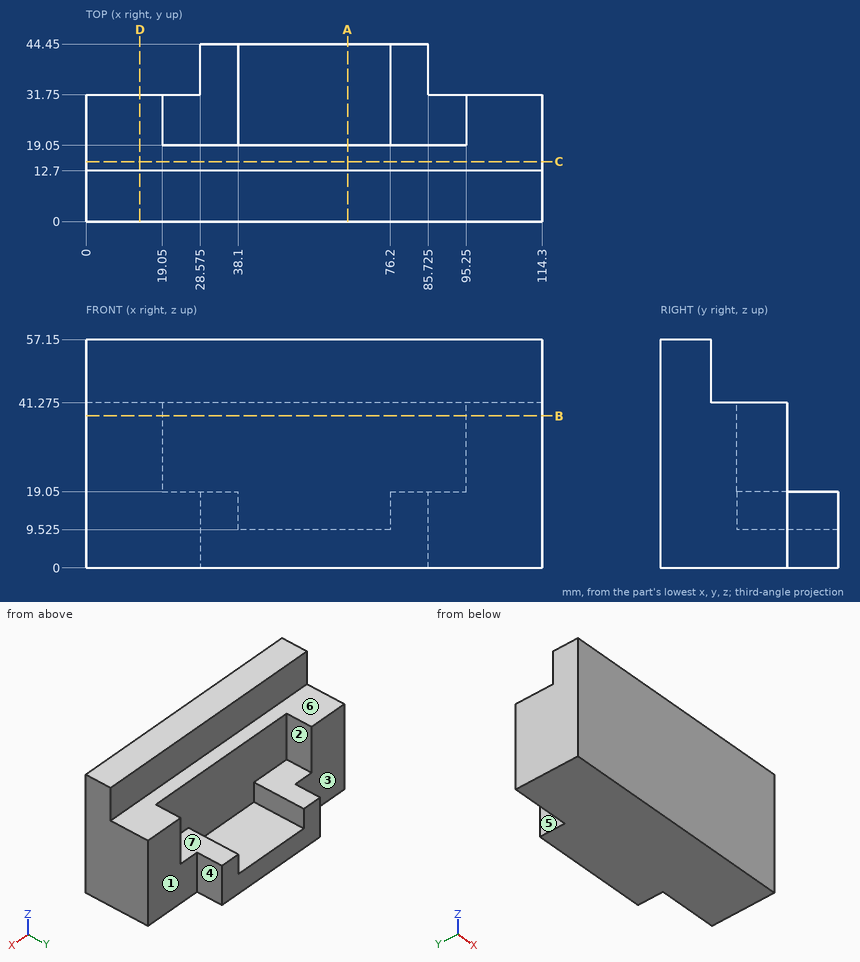
Drawing for the job (mm, zero at the part's lowest x, y, z). A direction names the side the tool comes from. Coordinates: 2 decimals unless noted, no trailing zeros. Order: outer loops, then holes, each group sorted by start corner. A loop starts at its lowest first (then second) coordinate and runs counter-clockwise, first axis right, second up. Notation, with made-up numbers: (13.5, 42.5) - (33.5, 42.5) arc R19 ccw to (33.5, 54.5) - close; hole circle Ø7 at (49, 41.5). An arc over 180 degrees is marked (long way). Use a Markdown table: item, result. Add a question column.
(1) Pull direction X, two halves, no side cores. Call the marked faces 4, 5, 6 and 7: +X half, -X half, draft (parallel to the pull), parting line (faces both ways), or undercut.
(2) Saw through at C-C (y = 15). Give the cut face in (x, z) (3 decimals).
(3) Saw through at D-D (x = 13.5). Give the cut face in (y, z) (3 decimals).
(4) Saw through at A-A (x = 65.5). Give the cut face in (y, z) (3 decimals), then the cut area to 3 significant figures.
(5) Drill centre lines: line 1 along X through (y, z) = (23.5, 16); line 2 along X through (y, z) = (22.5, 30); line 3 along Y through (x, z) = (25.5, 28). Where is each one in solid material? Low to high. Write a range as [from, to].
(6) Flat gauge pins, fed straight in: pin 1 (12 mm diameter, centred on x = 70, y = 36.5, fed in from +Z) (3 decimals); pin 2 (9.5 mm diameter, centred on x = 74, y = 22.5, fed in from +Z) (3 decimals); pin 3 (8.5 mm diameter, centred on x = 106, z = 24, fed in from +Y). Where does each tip first touch, or does it go through?
(7) Saw through at B-B (z = 38). Give the cut face in (x, y).
(8) Which spindle directions (+Z, -Z, +X, -X, +Y, -Y) get a long thin tool onto all of the face, cutting with end or side? Do the marked faces 1, 2 and 3. Say none if no direction does.
Solved:
| question | item | result |
|---|---|---|
| 1 | face 4 | +X half |
| 1 | face 5 | -X half |
| 1 | face 6 | draft |
| 1 | face 7 | undercut |
| 2 | outline | (0, 0) - (114.3, 0) - (114.3, 41.275) - (0, 41.275) - close |
| 3 | outline | (0, 0) - (31.75, 0) - (31.75, 41.275) - (12.7, 41.275) - (12.7, 57.15) - (0, 57.15) - close |
| 4 | outline | (0, 0) - (44.45, 0) - (44.45, 9.525) - (19.05, 9.525) - (19.05, 41.275) - (12.7, 41.275) - (12.7, 57.15) - (0, 57.15) - close |
| 4 | area | 1,230 mm² |
| 5 | line 1 | x = [0, 38.1], [76.2, 114.3] |
| 5 | line 2 | x = [0, 19.05], [95.25, 114.3] |
| 5 | line 3 | y = [0, 19.05] |
| 6 | pin 1 | stops at z = 9.525 |
| 6 | pin 2 | stops at z = 41.275 |
| 6 | pin 3 | stops at y = 31.75 |
| 7 | outline | (0, 0) - (114.3, 0) - (114.3, 31.75) - (95.25, 31.75) - (95.25, 19.05) - (19.05, 19.05) - (19.05, 31.75) - (0, 31.75) - close |
| 8 | face 1 | +Z, -Z, +X, +Y |
| 8 | face 2 | +Z, +Y |
| 8 | face 3 | +Z, -Z, -X, +Y |
